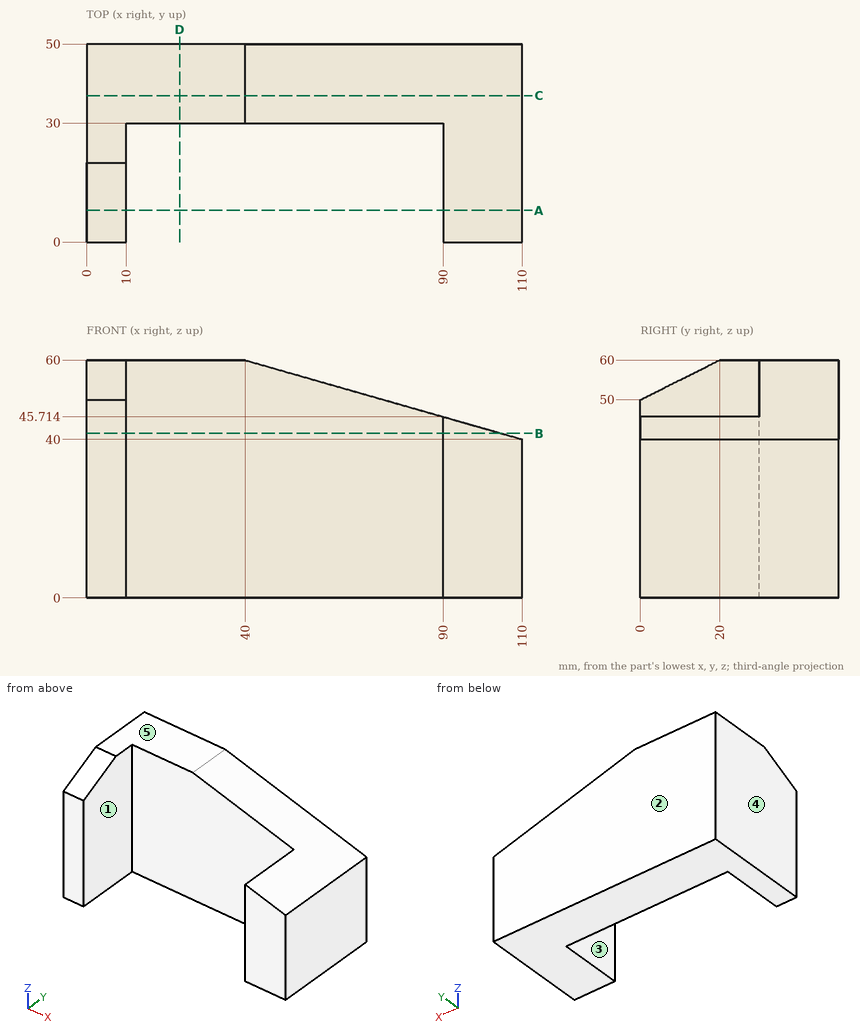
Input: dimensioned drawing with shaded views. Units: mm. Origin: part minimum x, y, z. A direction names the side the tool comes from. Give positions to 0.01 mm unless a question says otherwise; leave off trailing zeros. Write each loop counter-clockwise with the first axis right and the second up, starting at its lowest first coordinate (ties: lowest second). Pieces come first, ordered by that corner, then holes.
1. Pull-direction query (X, two-part tool) for the marked faces 3, 4 and 5; classes: +X half, -X half, draft (parallel to the pull), parting line (faces both ways), or undercut.
2. Material intervals for line 1 along X through (y, z) = (18.5, 17); line 2 along Y through (x, z) = (35.5, 13.5); line 3 along X through (y, z) = (28, 53), sorted ascending.
3. Section query C-C (y = 37). Return the cut outline in (x, z).
4. Section query D-D (x = 23.5). Return the cut outline in (y, z), then the cut area to 3 significant figures.
5. Section query B-B (z = 41.5). Return the cut outline in (x, y), then the cut area to 3 significant figures.
6. Section query A-A (y = 8). Return the cut outline in (x, z), then the cut area to 3 significant figures.
7. Access query for the marked faces 1 and 2. Directions: +Z, -Z, +X, -X, +Y, -Y. A direction counts if a zero-diameter tool reaches every point of the face in a straight line with its end or side. Return the directions, or none.
8. First-contact query: pin 1 (2 mm diameter, centred on x = 80, z = 27, fed in from -Y). Flat tip, straight axial feed; report the tip coordinate or a pass-through.
Output values:
1. face 3: undercut
1. face 4: -X half
1. face 5: draft
2. line 1: x = 0 to 10, 90 to 110
2. line 2: y = 30 to 50
2. line 3: x = 0 to 10
3. outline: (0, 0) - (110, 0) - (110, 40) - (40, 60) - (0, 60) - close
4. outline: (30, 0) - (50, 0) - (50, 60) - (30, 60) - close
4. area: 1,200 mm2
5. outline: (0, 0) - (10, 0) - (10, 30) - (90, 30) - (90, 0) - (104.75, 0) - (104.75, 50) - (0, 50) - close
5. area: 2,840 mm2
6. outline: (0, 0) - (10, 0) - (10, 54) - (0, 54) - close; (90, 0) - (110, 0) - (110, 40) - (90, 45.71) - close
6. area: 1,400 mm2
7. face 1: +Z, -Z, -Y
7. face 2: +Z, -Z, +X, -X, +Y
8. pin 1: stops at y = 30
